```python
from build123d import *

# Parameters (mm, degrees)
SKIZZE1_W                       = 123
SKIZZE1_H                       = 40
AUFSATZ_LINEAR_AUSTRAGEN1_DEPTH = 12.5
FASE_3X60_SIZE                  = 3
FASE_3X60_SIZE2                 = 5.196152423
FASE_5X45_SIZE                  = 5


with BuildPart() as part:
    # Skizze1 → Aufsatz-Linear austragen1 (new body, symmetric)
    with BuildSketch(Plane.XY):
        with Locations((61.5, 0)):
            Rectangle(SKIZZE1_W, SKIZZE1_H)
    extrude(amount=AUFSATZ_LINEAR_AUSTRAGEN1_DEPTH, both=True)

    # Skizze2 → Bohrung_Kegel 1_10 (revolve, cut)
    with BuildSketch(Plane(origin=(0, 0, 0), x_dir=(1, 0, 0), z_dir=(0, 1, 0)), mode=Mode.PRIVATE) as bohrung_kegel_1_10_sk:
        Polygon((103, -12.5), (87, -12.5), (87, -10), (94, -10), (93, 10), (87, 10), (87, 12.5), (103, 12.5), align=None)
    revolve(bohrung_kegel_1_10_sk.sketch.rotate(Axis((103, 0, 15.136672695), (0, 0, -1)), 180), axis=Axis((103, 0, 15.136672695), (0, 0, -1)), mode=Mode.SUBTRACT)  # turned: the seam where the file's is

    # Fase 3x60
    fase_3x60_edges = [part.edges().sort_by_distance(p)[0] for p in [
        (0, 20, 0),
        (0, -20, 0),
    ]]
    fase_3x60_side = [part.faces().sort_by_distance(p)[0] for p in [
        (0, 0, 0),
    ]]
    chamfer(fase_3x60_edges, length=FASE_3X60_SIZE, length2=FASE_3X60_SIZE2, reference=fase_3x60_side[0])

    # Fase 5x45
    fase_5x45_edges = [part.edges().sort_by_distance(p)[0] for p in [
        (123, 20, 0),
        (123, -20, 0),
    ]]
    chamfer(fase_5x45_edges, length=FASE_5X45_SIZE)


solid = part.part
```
Source: CAD feature listing. Evaluate the final solid. Frame: model axes, mm. A direction names the side the tool comes from. Coordinates: 2 decimals unless noted, no trailing zeros. Write each loop counter-clockwise with the first axis right and the second up, starting at its lowest first coordinate (ties: lowest second). Pieces come first, ordered by that corner, then holes. Notation, with made-up numbers: (62.25, 75.25) - (117.25, 75.25) arc R22 ccw to (117.25, 93.25) - close; hole circle Ø11 at (22, 5). An arc over 180 degrees is marked (long way). Answer as a JSON object with one key per item and string values.
Q1. Section query A-A, the plane x = 103. Output: boundary loops of the cut face in (y, z).
Ans:
{"outline": "(-20, -12.5) - (-16, -12.5) - (-16, -10) - (-10, -10) - (-9, 10) - (-16, 10) - (-16, 12.5) - (-20, 12.5) - close; (9, 10) - (10, -10) - (16, -10) - (16, -12.5) - (20, -12.5) - (20, 12.5) - (16, 12.5) - (16, 10) - close"}
Q2. Draft query along Y for faces 1 (the flat face through (2.6, 18.5, 0.2)), 2 (the conical face through (112.068, -2.856, -0.14)), 3 (the flat face through (61, -20, 0)). Return one class per face: released by +Y, released by -Y, zero draft, split by the parting line, or undercut.
Ans:
{"face 1": "released by +Y", "face 2": "undercut", "face 3": "released by -Y"}
Q3. Section query B-B, the plane y = 0. Output: boundary loops of the cut face in (x, z), plus the area to 4 significant figures.
Ans:
{"outline": "(0, -12.5) - (87, -12.5) - (87, -10) - (93, -10) - (94, 10) - (87, 10) - (87, 12.5) - (0, 12.5) - close; (112, 10) - (113, -10) - (119, -10) - (119, -12.5) - (123, -12.5) - (123, 12.5) - (119, 12.5) - (119, 10) - close", "area": "2,535 mm2"}
Q4. Section query C-C, the plane z = 5. Output: boundary loops of the cut face in (x, y).
Ans:
{"outline": "(0, -17) - (5.2, -20) - (118, -20) - (123, -15) - (123, 15) - (118, 20) - (5.2, 20) - (0, 17) - close; hole circle Ø18.5 at (103, 0)"}
Q5. Material intervals for line 1 (Y direction, x = 103, z = -10.75); line 2 (Y direction, x = 106.5, z = 6); line 3 (X direction, y = -5.5, z = 11.5), sorted ascending. Write a range as [from, to].
Ans:
{"line 1": "y = [-20, -16], [16, 20]", "line 2": "y = [-20, -8.51], [8.51, 20]", "line 3": "x = [0, 87.98], [118.02, 123]"}
Q6. Set-up query: faces 4 (the cylindrical face through (90.303, 9.736, -11.268)), 5 (the flat face through (0, 0, 0)), 6 (the flat face through (110, 7, 10)). Return all of +Z, -Z, +X, -X, +Y, -Y with unobstructed straight access to the full face (end or side cutting, diameter ignored); none if empty.
Ans:
{"face 4": "-Z", "face 5": "+Z, -Z, -X, +Y, -Y", "face 6": "+Z"}
Q7. First-contact query: pin 1 Ø16 at (x, y) = (103, 1.5) entering from +Z. Flat tip, straight axial feed; report the tip coordinate or a pass-through.
Ans:
{"pin 1": "stops at z = 10"}
Q8. Section query D-D, the plane z = -6. Output: boundary loops of the cut face in (x, y).
Ans:
{"outline": "(0, -17) - (5.2, -20) - (118, -20) - (123, -15) - (123, 15) - (118, 20) - (5.2, 20) - (0, 17) - close; hole circle Ø19.6 at (103, 0)"}
